Autodesk Inventor part; units mm, degrees
ref_plane "YZ Plane" through (0, 0, 0) normal (1, 0, 0) x (0, 1, 0)
ref_plane "XZ Plane" through (0, 0, 0) normal (0, 1, 0) x (-1, 0, 0)
ref_plane "XY Plane" through (0, 0, 0) normal (0, 0, 1) x (1, 0, 0)
sketch "Skizze1" plane through (0, 0, 0) normal (0, 1, 0) x (-1, 0, 0)
  line L0 (-19, 0) -> (-19, 30)
  line L1 (19, 30) -> (19, 0)
  line L2 (8.85, 11.45) -> (-8.85, 11.45)
  line L3 (-12.05, 11.45) -> (-12.05, 15.55)
  line L4 (-8.85, 15.55) -> (8.85, 15.55)
  line L5 (12.05, 15.55) -> (12.05, 11.45)
  arc A0 (12.05, 15.55) -> (8.85, 15.55) centre (10.45, 15.55) ccw
  arc A1 (8.85, 11.45) -> (12.05, 11.45) centre (10.45, 11.45) ccw
  arc A2 (-8.85, 15.55) -> (-12.05, 15.55) centre (-10.45, 15.55) ccw
  arc A3 (-12.05, 11.45) -> (-8.85, 11.45) centre (-10.45, 11.45) ccw
  line L6 (19, -3) -> (-19, -3)
  line L7 (-19, -3) -> (-19, 0)
  line L8 (19, 0) -> (19, -3)
  line L9 (0, 30) -> (19, 30)
  line L10 (19, 30) -> (-19, 30)
  arc A4 (-12.3, 11.45) -> (-8.617, 11.2) centre (-10.45, 11.45) ccw
  line L11 (-8.617, 11.2) -> (8.617, 11.2)
  arc A5 (8.617, 11.2) -> (12.3, 11.45) centre (10.45, 11.45) ccw
  line L12 (12.3, 11.45) -> (12.3, 15.55)
  arc A6 (12.3, 15.55) -> (8.617, 15.8) centre (10.45, 15.55) ccw
  line L13 (8.617, 15.8) -> (-8.617, 15.8)
  arc A7 (-8.617, 15.8) -> (-12.3, 15.55) centre (-10.45, 15.55) ccw
  line L14 (-12.3, 15.55) -> (-12.3, 11.45)
  line L15 (0, -3) -> (0, 30) construction
  point P0 (0, 13.5)
  point P1 (19, 0)
  point P2 (0, 13.5)
  dimension "d94" = 0.25
extrude "Grundkörper" add sketch "Skizze1" along normal mid plane 6 contours L0 L10 L9 L1 L8 L6 L7
sketch "Skizze10" plane through (19, 3, -3) normal (0, 0, -1) x (-1, 0, 0)
  line L0 (-3.4, -3) -> (41.4, -3)
  line L1 (19, 19.4) -> (19, -25.4)
  point P0 (19, -3)
  point P1 (19, -3)
  point P2 (3, -3)
  point P3 (35, -3)
  dimension "d96" = 32
hole "Fixierung" at (16, 0, -3) at (-16, 0, -3) direction (0, 0, 1) diameter 4.2 depth 8 tip angle 118
fillet "Rundung1" radius 1 2 edges at (-19, 0, 30) (19, 0, 30)
fillet "Rundung2" radius 0.2 4 edges at (-8.617, 0, 15.8) (8.617, 0, 15.8) (8.617, 0, 11.2) (-8.617, 0, 11.2)
sketch "Skizze13" plane through (0, -3, 0) normal (0, -1, 0) x (1, 0, 0)
  line L0 (-8.6611, 15.55) -> (8.6611, 15.55) construction
  line L1 (0, 15.55) -> (0, 11.45) construction
  line L2 (-8.6611, 11.45) -> (8.6611, 11.45) construction
  line L3 (-11.8, 6.7) -> (11.8, 6.7)
  line L4 (13.8, 8.7) -> (13.8, 18.3)
  line L5 (11.8, 20.3) -> (-11.8, 20.3)
  line L6 (-13.8, 18.3) -> (-13.8, 8.7)
  line L7 (-13.8, 6.7) -> (13.8, 20.3) construction
  line L8 (13.8, 6.7) -> (-13.8, 20.3) construction
  arc A0 (-11.8, 20.3) -> (-13.8, 18.3) centre (-11.8, 18.3) ccw
  arc A1 (-13.8, 8.7) -> (-11.8, 6.7) centre (-11.8, 8.7) ccw
  arc A2 (11.8, 6.7) -> (13.8, 8.7) centre (11.8, 8.7) ccw
  arc A3 (13.8, 18.3) -> (11.8, 20.3) centre (11.8, 18.3) ccw
  point P0 (0, 0)
  point P1 (0, 13.5)
  dimension "d125" = 27.6
  dimension "d126" = 13.6
  dimension "d127" = 2
extrude "Tasche" cut sketch "Skizze13" against normal blind 1
sketch "Skizze11" plane through (19, -3, -3) normal (1, 0, 0) x (0, 0, -1)
  point P0 (-7, 3)
  point P1 (-17, 3)
hole "Federn" at (19, 0, 14) direction (-1, 0, 0) diameter 2 depth 4 tip angle 118
mirror "Spiegeln1" about plane through (0, 0, 0) normal (1, 0, 0) of "Federn"
sketch "Skizze12" plane through (-18, 3, 30) normal (0, 0, 1) x (1, 0, 0)
  line L0 (18, -3) -> (2, -3)
  line L1 (18, -3) -> (18, 0)
  line L2 (26.6611, 0) -> (9.3389, 0)
  point P0 (34, -3)
  dimension "d117" = 16
hole "Platinenhalterung" at (-16, 0, 30) at (16, 0, 30) direction (0, 0, -1) diameter 4.1 depth 8 tip angle 118
properties part number "Spulenhalter Hinten Einzel" material "Aluminium 6061"
The listing builds one solid part. Answer for the finished solid, in the listing's coordinates (mm). A direction names the side the tool comes from. Give positions to 0.01 mm unless a question says otherwise; leave off trailing zeros. Write each loop counter-clockwise with the first axis right and the second up, starting at its lowest first coordinate (ties: lowest second). Pieces come first, ordered by that corner, then holes.
1) Section B-B (z = 4) is taken. Write down the section's boundary in (x, y).
2) Given P1, Ø11, axis at x = 6.5, z = 14, coming from the -Y side; P2, Ø3.5, axis at x = -16, y = 0, coming from the -Z side; P3, Ø1.8, axis at y = 0, z = 14, coming from the -X side, each flat-ended and moving along its own axis, determine where each tip first touches the part or whether it passes through.
3) Find the intervals of material crossed by L1, parallel to X at y = 0, z = -1; L2, parallel to Z at x = 7.5, y = -1; L3, parallel to Y at x = -16.9, z = 14, in increasing order.
4) For a pull along Y with two mould halves and no side action, classify faces 1 (the face through (0, -2, 17)), 2 (the face through (-16.36, -0.08, 6.04)), 3 (the face through (13.23, -2.51, 19.7)) as pulls with the +Y half, pulls with the -Y half, needs draft (parallel to the pull), parting line crosses it, or undercut.
5) Section C-C (z = 27) is taken. Write down the section's boundary in (x, y).
6) A tool of negligible diameter and unlimited length cuts with its end or side. For faces 4 (the face through (-17.77, 1.13, 1.06)), 5 (the face through (0.2, -2.5, 20.3)), 6 (the face through (10.692, 0.465, 17.384)), from which of +Z, -Z, +X, -X, +Y, -Y can it reach the whole face along a straight path? Write none if from no direction.
7) Section A-A (x = 2.5) is taken. Write down the section's boundary in (y, z).
Response:
1. outline: (-19, -3) - (19, -3) - (19, 3) - (-19, 3) - close; hole circle Ø4.2 at (-16, 0); hole circle Ø4.2 at (16, 0)
2. P1: stops at y = -2
2. P2: stops at z = 5.21
2. P3: stops at x = -14.94
3. L1: x = -19 to -18.1, -13.9 to 13.9, 18.1 to 19
3. L2: z = -3 to 11.2, 15.8 to 30
3. L3: y = -3 to -1, 1 to 3
4. face 1: pulls with the -Y half
4. face 2: undercut
4. face 3: needs draft
5. outline: (-19, -3) - (19, -3) - (19, 3) - (-19, 3) - close; hole circle Ø4.1 at (-16, 0); hole circle Ø4.1 at (16, 0)
6. face 4: -Z
6. face 5: -Y
6. face 6: +Y, -Y
7. outline: (-3, -3) - (3, -3) - (3, 11.2) - (-2, 11.2) - (-2, 6.7) - (-3, 6.7) - close; (-3, 20.3) - (-2, 20.3) - (-2, 15.8) - (3, 15.8) - (3, 30) - (-3, 30) - close
